Source: CAD feature listing. Evaluate the final solid. Frame: model axes, mm. A direction names the side the tool comes from. Give positions to 0.01 mm unless a question says otherwise; leave off trailing zeros. Loops run counter-clockwise (first coordinate to the right, second up) from the corner with the lowest first, then second, coordinate; pieces in that order, holes last. Notation, with made-up numbers: M -22,19.5 L 21,19.5 A28 cw 21,49.5 Z; hole C -16,24.25 d6. An arc over 180 degrees is marked long. Put each result on its own line as item: value.
from build123d import *

# Parameters (mm, degrees)
BOX014_W              = 5.2
BOX014_H              = 15
BOX014_DEPTH          = 67
FILLET001_R           = 2.55
BOX021_W              = 17
BOX021_H              = 40
BOX021_DEPTH          = 24
CYLINDER005_R         = 3.2
CYLINDER005_DEPTH     = 4
CYLINDER007_R         = 1.9
CYLINDER007_DEPTH     = 6
CYLINDER006_R         = 1.65
CYLINDER006_DEPTH     = 54
BOX006_W              = 17
BOX006_H              = 42
BOX006_DEPTH          = 40
CHAMFER020026003_SIZE = 9


with BuildPart() as fillet001:
    # Box014 → Box014 (new body)
    with BuildSketch(Plane(origin=(6.4, 15, -6), x_dir=(1, 0, 0), z_dir=(0, 0, 1))):
        with Locations((2.6, 7.5)):
            Rectangle(BOX014_W, BOX014_H)
    extrude(amount=BOX014_DEPTH)

    # Fillet001
    fillet001_edges = [fillet001.edges().sort_by_distance(p)[0] for p in [
        (6.4, 15, 27.5),
        (6.4, 30, 27.5),
        (11.6, 15, 27.5),
        (11.6, 30, 27.5),
    ]]
    fillet(fillet001_edges, radius=FILLET001_R)


with BuildPart() as cube021:
    # Box021 → Box021 (new body)
    with BuildSketch(Plane(origin=(0, 10, 2), x_dir=(1, 0, 0), z_dir=(0, 0, 1))):
        with Locations((8.5, 20)):
            Rectangle(BOX021_W, BOX021_H)
    extrude(amount=BOX021_DEPTH)


with BuildPart() as cylinder005:
    # Cylinder005 → Cylinder005 (new body)
    with BuildSketch(Plane(origin=(9, 39, 31), x_dir=(1, 0, 0), z_dir=(0, 0, 1))):
        Circle(CYLINDER005_R)
    extrude(amount=CYLINDER005_DEPTH)


with BuildPart() as cylinder007:
    # Cylinder007 → Cylinder007 (new body)
    with BuildSketch(Plane(origin=(9, 39, -6), x_dir=(1, 0, 0), z_dir=(0, 0, 1))):
        Circle(CYLINDER007_R)
    extrude(amount=CYLINDER007_DEPTH)


with BuildPart() as cylinder006:
    # Cylinder006 → Cylinder006 (new body)
    with BuildSketch(Plane(origin=(9, 39, -12), x_dir=(1, 0, 0), z_dir=(0, 0, 1))):
        Circle(CYLINDER006_R)
    extrude(amount=CYLINDER006_DEPTH)


with BuildPart() as cut002002002007004004001006016:
    # Box006 → Box006 (new body)
    with BuildSketch(Plane(origin=(0, 3, -6), x_dir=(1, 0, 0), z_dir=(0, 0, 1))):
        with Locations((8.5, 21)):
            Rectangle(BOX006_W, BOX006_H)
    extrude(amount=BOX006_DEPTH)

    # Chamfer020026003
    chamfer020026003_edges = [cut002002002007004004001006016.edges().sort_by_distance(p)[0] for p in [
        (17, 45, 14),
    ]]
    chamfer(chamfer020026003_edges, length=CHAMFER020026003_SIZE)

    # Cut002002002007004004001006009: cut Cylinder006
    add(cylinder006.part, mode=Mode.SUBTRACT)

    # Cut002002002007004004001006010: cut Cylinder007
    add(cylinder007.part, mode=Mode.SUBTRACT)

    # Cut002002002007004004001006011: cut Cylinder005
    add(cylinder005.part, mode=Mode.SUBTRACT)

    # Cut002002002007004004001006012: cut Cube021
    add(cube021.part, mode=Mode.SUBTRACT)

    # Cut002002002007004004001006016: cut Fillet001
    add(fillet001.part, mode=Mode.SUBTRACT)


solid = cut002002002007004004001006016.part
1. Material intervals for line 1 (Z direction, x = 4, y = 30); line 2 (Y direction, x = 9, z = 32.05); line 3 (Y direction, x = 9, z = -3.95), sorted ascending. Write a range as from..to.
Found:
line 1: -6..2, 26..34
line 2: 3..15, 30..35.8, 42.2..44
line 3: 3..15, 30..37.1, 40.9..44
2. Section query D-D (x = 10). State how many separate pieces and enclosed holes the cut face has, plus the area to 3 significant figures.
Found:
separate pieces: 5
enclosed holes: 0
area: 518 mm^2
3. Section query A-A (y = 39). Output: boundary loops of the cut face in (x, z).
Found:
outline: M 0,-6 L 7.1,-6 L 7.1,0 L 7.35,0 L 7.35,2 L 0,2 Z; M 0,26 L 7.35,26 L 7.35,31 L 5.8,31 L 5.8,34 L 0,34 Z; M 10.65,0 L 10.9,0 L 10.9,-6 L 14,-6 L 14,2 L 10.65,2 Z; M 10.65,26 L 14,26 L 14,34 L 12.2,34 L 12.2,31 L 10.65,31 Z
4. Access query for faces 5 (the flat face through (5, 28, 2)), 6 (the cylindrical face through (10.833, 15.727, 30.056)), 7 (the flat face through (10.4, 37.6, 31)). Directions: +Z, -Z, +X, -X, +Y, -Y. A direction counts if a zero-diameter tool reaches every point of the face in a straight line with its end or side. Return the directions, or none.
Found:
face 5: +X, -X, +Y
face 6: +Z, -Z
face 7: +Z
5. Section query C-C (y = 34). Output: boundary loops of the cut face in (x, z).
Found:
outline: M 0,-6 L 17,-6 L 17,2 L 0,2 Z; M 0,26 L 17,26 L 17,34 L 0,34 Z
6. Draft query along Y for faces 1 (the cylindrical face through (7.127, 29.233, -1.944)), 2 (the flat face through (5, 24, -6)), 3 (the cylindrical face through (9.89, 40.39, 28.47)), 4 (the flat face through (12, 41, -2)). Return one class per face: pulls with the +Y half, pulls with the -Y half, needs draft (parallel to the pull), parting line crosses it, or undercut.
Found:
face 1: undercut
face 2: needs draft
face 3: undercut
face 4: pulls with the +Y half
7. Section query B-B (z = 27). Output: boundary loops of the cut face in (x, y), plus the area to 3 significant figures.
Found:
outline: M 0,3 L 17,3 L 17,36 L 8,45 L 0,45 Z; hole M 6.4,17.55 A2.55 ccw 8.95,15 L 9.05,15 A2.55 ccw 11.6,17.55 L 11.6,27.45 A2.55 ccw 9.05,30 L 8.95,30 A2.55 ccw 6.4,27.45 Z; hole C 9,39 d3.3
area: 593 mm^2
8. Contact query for flat-ended pins moving along their axis: P1, Ø1.5, axis at x = 2.5, z = 25, coming from the +Y side; P2, Ø2.5, axis at x = 9, y = 39, coming from the -Z side; P3, Ø3.5, axis at x = 9, y = 39, coming from the +Z side. Output: stop coordinate, or through.
Found:
P1: y = 10
P2: through
P3: z = 31
